Part model, mm, in its own coordinate system. A direction names the side the tool comes from. Give positions to 0.01 mm unless a question says otherwise; leave off trailing zeros. Order: outer loops, then holes, each group sorted by start corner. A loop starts at its lowest first (then second) coordinate and runs counter-clockwise, first axis right, second up. Notation, with made-up numbers: M -32,48 L -14,48 A38 ccw -14,87 Z; hole C -19.5,84.5 d2. An arc over 180 degrees is marked long. Return JSON: item names as keys, results as strings.
from build123d import *

# Parameters (mm, degrees)
F1_DEPTH = 25
F2_T     = 2
F3_R     = 9.8912008391
F3_R_2   = 4.387511957
F3_R_3   = 6.4247632348
F4_DEPTH = 25


with BuildPart() as f1:
    # F0 (on Top) → F1 (new body)
    with BuildSketch(Plane.XY):
        Polygon((23.0428799987, 34.2442803085), (0, 58.5673190653), (-20.1625209302, 34.2442803085), (-5.1206401549, 34.2442803085), (-29.7637209296, 11.2014003098), (-5.1206401549, 11.2014003098), (-40.0050021708, -16.6420806199), (-5.1206401549, -16.6420806199), (-5.1206401549, -35.5244390666), (5.1206401549, -35.5244390666), (5.1206401549, -16.6420806199), (34.2442803085, -16.6420806199), (5.1206401549, 11.2014003098), (29.1236396879, 11.2014003098), (5.0213176084, 34.2442803085), align=None)
    extrude(amount=F1_DEPTH)

    # F2
    f2_openings = [f1.faces().sort_by_distance(p)[0] for p in [
        (-0.665195, 9.585773, 25),
    ]]
    offset(amount=F2_T, openings=f2_openings, kind=Kind.INTERSECTION)

    # F3 (on face) → F4 (cut)
    with BuildSketch(Plane(origin=(0, 0, -2), x_dir=(1, 0, 0), z_dir=(0, 0, -1))):
        Circle(F3_R)
        with Locations((0, -46.9125165525)):
            Circle(F3_R_2)
        with Locations((0, -28.6650005728)):
            Circle(F3_R_3)
    extrude(amount=-F4_DEPTH, mode=Mode.SUBTRACT)


solid = f1.part
Q1. Probe line 1 along Y through (x, z) = (-23, 20); line 2 along X through (y, z) = (-23, 8); line 3 along Y through (x, z) = (0, -0.95) (3 decimals). List the from-to ranges inside material, lowest first.
Established:
{"line 1": "y = -18.64 to -16.64, -3.07 to -0.51, 9.2 to 11.2, 17.53 to 20.26, 32.24 to 33.96", "line 2": "x = -7.12 to -5.12, 5.12 to 7.12", "line 3": "y = -37.524 to -9.891, 9.891 to 22.24, 35.09 to 42.525, 51.3 to 61.475"}
Q2. Band-saw the part on C-C (x = 19). Give the cut face in (y, z), then the cut area to 3 significant figures.
Established:
{"outline": "M -18.64,-2 L 0.7,-2 L 0.7,25 L -2.07,25 L -2.07,0 L -16.64,0 L -16.64,25 L -18.64,25 Z; M 9.2,-2 L 23.65,-2 L 23.65,25 L 20.88,25 L 20.88,0 L 11.2,0 L 11.2,25 L 9.2,25 Z; M 32.24,-2 L 41.42,-2 L 41.42,25 L 38.51,25 L 38.51,0 L 34.24,0 L 34.24,25 L 32.24,25 Z", "area": "447 mm²"}
Q3. Two-plate mould, pull along X, no slides. Class faces 1 (the flat face through (7.121, -28, 11)), 2 (the flat face through (-9.94, 46.576, 12.325)), 3 (the flat face through (-28, -4.5, 11.3)): +X half, -X half, draft (parallel to the pull), parting line (faces both ways), or undercut.
Established:
{"face 1": "+X half", "face 2": "undercut", "face 3": "-X half"}
Q4. 3-axis set-ups, long thin cutter, end or side, ignore diameter. For faces 4 (the flat face through (-12.089, 47.118, 11.311)), 5 (the flat face through (0, 12, -2)), 6 (the flat face through (19.89, -2.92, 12.32)), 7 (the flat face through (-7.121, -28, 11)), 8 (the flat face through (24.872, -4.915, 11.311)): which of +Z, -Z, +X, -X, +Y, -Y reach the whole face in a straight line?
Established:
{"face 4": "+Z, -Z, -X, +Y", "face 5": "-Z, +X, -X, +Y, -Y", "face 6": "+Z", "face 7": "+Z, -Z, -X, -Y", "face 8": "+Z, -Z, +X"}
Q5. Band-saw the part on D-D (y = 0). Give the cut face in (x, z), then the cut area to 3 significant figures.
Established:
{"outline": "M -22.36,-2 L -9.89,-2 L -9.89,0 L -19.15,0 L -19.15,25 L -22.36,25 Z; M 9.89,-2 L 19.73,-2 L 19.73,25 L 16.84,25 L 16.84,0 L 9.89,0 Z", "area": "197 mm²"}
Q6. Pin check, flat tips, straight feed: pin 1 (1.5 mm diameter, centred on y = 24.5, z = 5.5, fed in from -X); pin 2 (4 mm diameter, centred on y = -15.5, z = 15.5, fed in from +X); pin 3 (7 mm diameter, centred on x = -16, z = 14.5, fed in from -Y); pin 4 (10 mm diameter, centred on x = -35.5, y = -24.5, fed in from +Z). Stop position of each tip, or through.
Established:
{"pin 1": "stops at x = -19.27", "pin 2": "stops at x = 38.04", "pin 3": "stops at y = -18.64", "pin 4": "passes through"}
Q7. Band-saw the part on B-B (y = -22). Give the cut face in (x, z), then the cut area to 3 significant figures.
Established:
{"outline": "M -7.12,-2 L 7.12,-2 L 7.12,25 L 5.12,25 L 5.12,0 L -5.12,0 L -5.12,25 L -7.12,25 Z", "area": "128 mm²"}
